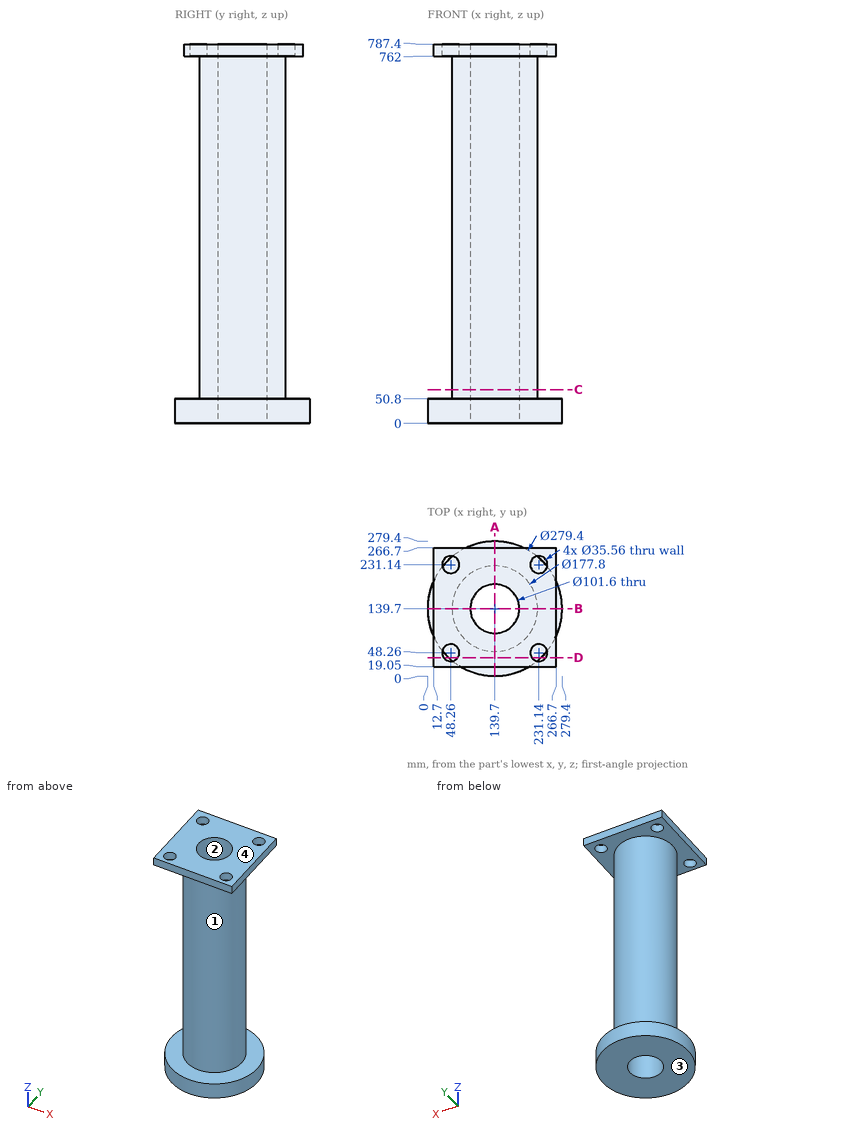
Geometry check sheet. Reference: drawing and pictorial views, mm from the part's lowest x, y, z. Give positions to 0.01 mm unless a question says otherwise; leave off trailing zeros. Write each loop counter-clockwise with the first axis right and the second up, starting at its lowest first coordinate (ties: lowest second). Pieces come first, ordered by that corner, then holes. Notation, with made-up numbers: (-34.5, 21) -> (16.5, 21) arc R23 ccw to (16.5, 60) -> close; hole circle Ø7 at (83, -8). An arc over 180 degrees is marked (long way). One line per item, written item: value. Start each with the question number.
Item 1: Material ranges on probe 1 along Y at (x, z) = (231.14, 782.5); probe 2 along X at (y, z) = (48, 775); probe 3 along Z at (x, y) = (238, 114), recorded low to high. Write a range as from..to.
Item 2: Section check D-D on y = 38. Record the cut outline in (x, z).
Item 3: Gauge pin test, flat ends, axial feed: pin 1 (12.5 mm diameter, centred on y = 95.5, z = 771, fed in from -X); pin 2 (5 mm diameter, centred on y = 110.5, z = 206, fed in from -X); pin 3 (21.5 mm diameter, centred on x = 48.26, y = 48.26, fed in from +Z). Record the tip position at first contact, or that the pin passes through.
Item 4: Section check B-B on y = 139.7. Record the cut outline in (x, z), then the cut area to 3 significant figures.
Item 5: Section check A-A on x = 139.7. Record the cut outline in (y, z), then the cut area to 3 significant figures.
Item 6: Section check C-C on z = 70. Record the cut outline in (x, y), then the cut area to 3 significant figures.
Item 7: Draft check along Z on the marked faces 1, 2, 3 and 4. Enter one of: +Z half, -Z half, draft (parallel to the pull), parting line (faces both ways), or undercut.
Results list:
1. probe 1: 19.05..30.48, 66.04..213.36, 248.92..266.7
1. probe 2: 12.7..30.48, 66.04..213.36, 248.92..266.7
1. probe 3: 0..50.8, 762..787.4
2. outline: (12.7, 762) -> (33.74, 762) -> (33.74, 787.4) -> (12.7, 787.4) -> close; (43.92, 0) -> (235.48, 0) -> (235.48, 50.8) -> (43.92, 50.8) -> close; (62.78, 762) -> (216.62, 762) -> (216.62, 787.4) -> (62.78, 787.4) -> close; (245.66, 762) -> (266.7, 762) -> (266.7, 787.4) -> (245.66, 787.4) -> close
3. pin 1: x = 12.7
3. pin 2: x = 54.9
3. pin 3: z = 50.8
4. outline: (0, 0) -> (88.9, 0) -> (88.9, 787.4) -> (12.7, 787.4) -> (12.7, 762) -> (50.8, 762) -> (50.8, 50.8) -> (0, 50.8) -> close; (190.5, 0) -> (279.4, 0) -> (279.4, 50.8) -> (228.6, 50.8) -> (228.6, 762) -> (266.7, 762) -> (266.7, 787.4) -> (190.5, 787.4) -> close
4. area: 67,100 mm²
5. outline: (0, 0) -> (88.9, 0) -> (88.9, 787.4) -> (19.05, 787.4) -> (19.05, 762) -> (50.8, 762) -> (50.8, 50.8) -> (0, 50.8) -> close; (190.5, 0) -> (279.4, 0) -> (279.4, 50.8) -> (228.6, 50.8) -> (228.6, 762) -> (266.7, 762) -> (266.7, 787.4) -> (190.5, 787.4) -> close
5. area: 66,900 mm²
6. outline: circle Ø177.8 at (139.7, 139.7); hole circle Ø101.6 at (139.7, 139.7)
6. area: 16,700 mm²
7. face 1: undercut
7. face 2: draft
7. face 3: -Z half
7. face 4: +Z half
